For this review, take the finished solid that the model builds, in its own axes (mm). Face numbers are marked on the shaded views. A direction names the side the tool comes from. Round coordinates to 2 decimals unless told otherwise and drop trailing zeros. Order: outer loops, then holes, each group sorted by start corner. A loop starts at its lowest first (then second) coordinate and runs counter-clockwise, first axis right, second up. Notation, with made-up numbers: M 55.25,20.5 L 110.25,20.5 A28 ccw 110.25,42.5 Z; hole C 53,-39 d9. An arc over 180 degrees is marked long. Put each result on its own line as item: value.
Autodesk Fusion 360 part; units mm, degrees
sketch "Sketch1" plane through (0, 0, 0) normal (0, 0, 1) x (1, 0, 0)
  line L0 (20, 0) -> (130, 0)
  line L1 (150, 20) -> (150, 110)
  line L2 (130, 130) -> (20, 130)
  line L3 (0, 110) -> (0, 20)
  arc A0 (20, 130) -> (0, 110) centre (20, 110) ccw
  arc A1 (150, 110) -> (130, 130) centre (130, 110) ccw
  arc A2 (130, 0) -> (150, 20) centre (130, 20) ccw
  arc A3 (0, 20) -> (20, 0) centre (20, 20) ccw
  point P0 (150, 0)
  point P1 (0, 130)
  dimension "d1" = 150
  dimension "d2" = 130
  dimension "d3" = 20
extrude "Extrude1" add sketch "Sketch1" along normal blind 7.5
sketch "Sketch2" plane through (0, 0, 7.5) normal (0, 0, 1) x (-1, 0, 0)
  arc A0 (0, -20) -> (-20, 0) centre (-20, -20) ccw
  line L0 (-20, 0) -> (-130, 0)
  arc A1 (-130, 0) -> (-150, -20) centre (-130, -20) ccw
  line L1 (-150, -20) -> (-150, -110)
  arc A2 (-150, -110) -> (-130, -130) centre (-130, -110) ccw
  line L2 (-130, -130) -> (-20, -130)
  arc A3 (-20, -130) -> (0, -110) centre (-20, -110) ccw
  line L3 (0, -110) -> (0, -20)
  line L4 (-75, -130) -> (-75, 0) construction
  line L5 (0, -65) -> (-150, -65) construction
  line L6 (-115, -58.75) -> (-35, -58.75) construction
  line L7 (-35, -58.75) -> (-35, -71.25) construction
  line L8 (-35, -71.25) -> (-115, -71.25) construction
  line L9 (-115, -71.25) -> (-115, -58.75) construction
  line L10 (-115, -58.75) -> (-35, -71.25) construction
  line L11 (-35, -58.75) -> (-115, -71.25) construction
  line L12 (-35, -65) -> (-60, -65) construction
  line L13 (-60, -65) -> (-60, -75)
  line L14 (-60, -75) -> (-25, -75)
  line L15 (-60, -65) -> (-60, -55)
  line L16 (-60, -55) -> (-25, -55)
  line L17 (-25, -55) -> (-25, -75)
  point P0 (-75, -65)
  dimension "d6" = 80
  dimension "d7" = 12.5
  dimension "d10" = 25
  dimension "d11" = 10
  dimension "d12" = 10
extrude "Extrude2" add sketch "Sketch2" along normal blind 30 contours L13 L14 L15 L16 L17
sketch "Sketch3" plane through (0, 0, 37.5) normal (0, 0, 1) x (-1, 0, 0)
  line L0 (-60, -55) -> (-60, -75)
  line L1 (-60, -75) -> (-25, -75)
  line L2 (-25, -75) -> (-25, -55)
  line L3 (-25, -55) -> (-60, -55)
  line L4 (-60, -65) -> (-35, -65) construction
  line L5 (-35, -65) -> (-40, -65) construction
  circle A0 centre (-40, -65) radius 2.5
  circle A1 centre (-55, -65) radius 2.5
  dimension "d15" = 5
  dimension "d18" = -15
  dimension "d19" = 0
extrude "Extrude3" cut sketch "Sketch3" against normal blind 37.5 contours A0 | A1
sketch "Sketch4" plane through (0, 0, 0) normal (0, 0, -1) x (1, 0, 0)
  circle A0 centre (40, -65) radius 2.5
  circle A1 centre (55, -65) radius 2.5
  arc A2 (20, 0) -> (0, -20) centre (20, -20) ccw
  line L0 (0, -20) -> (0, -110)
  arc A3 (0, -110) -> (20, -130) centre (20, -110) ccw
  line L1 (20, -130) -> (130, -130)
  arc A4 (130, -130) -> (150, -110) centre (130, -110) ccw
  line L2 (150, -110) -> (150, -20)
  arc A5 (150, -20) -> (130, 0) centre (130, -20) ccw
  line L3 (130, 0) -> (20, 0)
  circle A6 centre (40, -65) radius 5
  circle A7 centre (55, -65) radius 5
  dimension "d22" = 10
  dimension "d23" = 10
extrude "Extrude4" cut sketch "Sketch4" against normal blind 7.5 contours A6 | A7
fillet "Fillet1" radius 7 6 edges at (25, 65, 7.5) (42.5, 55, 7.5) (25, 55, 22.5) (25, 75, 22.5) (25, 65, 37.5) (42.5, 75, 7.5)
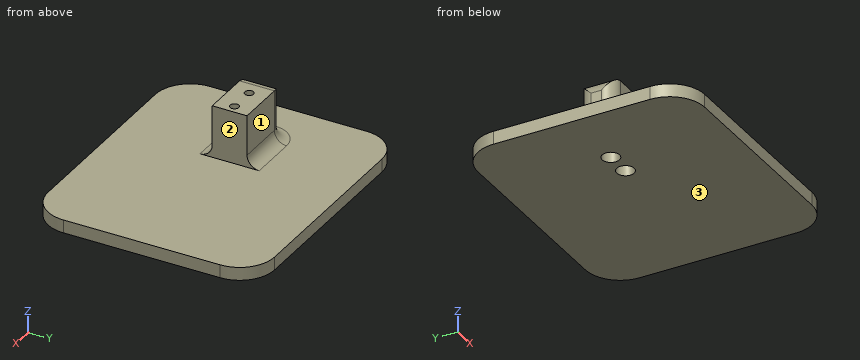
(1) Add section B-B on z = 21.5. Give the boundary of the cut face in (x, y).
A:
outline: M 25,62 A7 ccw 32,55 L 60,55 L 60,75 L 32,75 A7 ccw 25,68 Z; hole C 40,65 d5; hole C 55,65 d5
(2) Insertion check: pin 1 Ø7 at (x, z) = (43.5, 25) entering from -Y; pin 2 Ø1.5 at (x, y) = (106.5, 80) entering from +Z; pin 3 Ø5 at (y, z) = (73.5, 14) entering from +X. Each pin has a flat end and moves straight along its axis. Give the tip position at first contact, or say it passes through.
A:
pin 1: stops at y = 55
pin 2: stops at z = 7.5
pin 3: stops at x = 60
(3) Add section C-C on y = 35.5. Give the boundary of the cut face in (x, z), then the cut area to 4 significant figures.
A:
outline: M 0,0 L 150,0 L 150,7.5 L 0,7.5 Z
area: 1,125 mm2
(4) To check wall thickness, follow L1, parallel to X at y = 65, z = 21.75; L2, parallel to X at y = 65, z = 4; L3, parallel to Y at x = 40, z = 19.25. State the ranges of each line that lie inside material, in increasing order.
A:
L1: x = 25 to 37.5, 42.5 to 52.5, 57.5 to 60
L2: x = 0 to 35, 45 to 50, 60 to 150
L3: y = 55 to 62.5, 67.5 to 75
(5) Add section D-D on x = 70.5. Give the boundary of the cut face in (y, z), then the cut area to 3 significant figures.
A:
outline: M 0,0 L 130,0 L 130,7.5 L 0,7.5 Z
area: 975 mm2
(6) For the marked faces 1, 2 and 3, list the 3-axis set-ups (+Z, -Z, +X, -X, +Y, -Y) from which the entire face can be reached by the end or side of a thin tool; tool diameter is ignored.
A:
face 1: +Z, +X, -X, +Y
face 2: +Z, +X, +Y, -Y
face 3: -Z, +X, -X, +Y, -Y
(7) Add section A-A on x = 55. Give the boundary of the cut face in (y, z).
A:
outline: M 0,0 L 60,0 L 60,7.5 L 62.5,7.5 L 62.5,37.5 L 55,37.5 L 55,14.5 A7 cw 48,7.5 L 0,7.5 Z; M 67.5,7.5 L 70,7.5 L 70,0 L 130,0 L 130,7.5 L 82,7.5 A7 cw 75,14.5 L 75,37.5 L 67.5,37.5 Z
